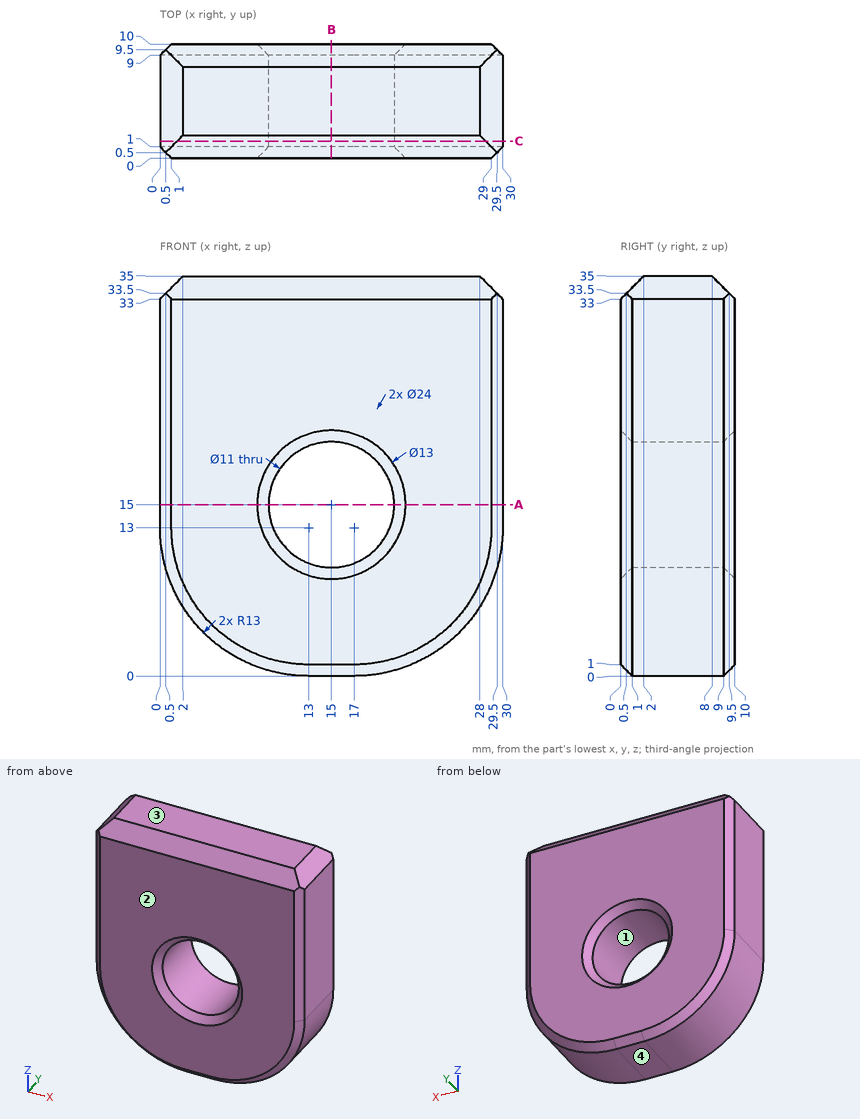
Job drawing, mm, ordinate dimensions from the low corner. One solid piece. Give positions to 0.01 mm unless a question says otherwise; leave off trailing zeros. Loops run counter-clockwise (first coordinate to the right, second up) from the corner with the lowest first, then second, coordinate; pieces in that order, holes last. Notation, with made-up numbers: (-19, 58.25) -> (3, 58.25) arc R25 cw to (3, 71.25) -> close; hole circle Ø3 at (85, 38). An arc over 180 degrees is marked (long way). Use a Markdown table: item, result. Add a question column.
(1) Wall check: line 1 along Z through (x, y) = (15, 3.75); line 2 along X through (y, z) = (4.5, 11.5); line 3 along X through (y, z) = (1.5, 17). Give the ranges that are in metal, low to high.
(2) Slice it at A-A on z = 15. List the corners of the cut face in (x, y).
(3) Mould opens along Z. For the marked faces 1, 2, 3 and 4 say: +Z half, -Z half, draft (parallel to the pull), parting line (faces both ways), or undercut.
(4) Slice it at B-B on x = 15. List the corners of the cut face in (y, z), and give its area (3 significant figures).
(5) Drop a flat-ended pin along its axis: pin 1 Ø1 at (y, z) = (3.5, 5.5) entering from +X. Give the stop position or say it passes through.
(6) Slice it at C-C on y = 1.5. List the corners of the cut face in (x, z).
Filled sheet:
| question | item | result |
|---|---|---|
| 1 | line 1 | 0 to 9.5, 20.5 to 35 |
| 1 | line 2 | 0.09 to 10.76, 19.24 to 29.91 |
| 1 | line 3 | 0 to 9.88, 20.12 to 30 |
| 2 | outline | (0, 1) -> (1, 0) -> (8.5, 0) -> (9.5, 1) -> (9.5, 9) -> (8.5, 10) -> (1, 10) -> (0, 9) -> close; (20.5, 1) -> (21.5, 0) -> (29, 0) -> (30, 1) -> (30, 9) -> (29, 10) -> (21.5, 10) -> (20.5, 9) -> close |
| 3 | face 1 | undercut |
| 3 | face 2 | draft |
| 3 | face 3 | +Z half |
| 3 | face 4 | -Z half |
| 4 | outline | (0, 1) -> (1, 0) -> (9, 0) -> (10, 1) -> (10, 8.5) -> (9, 9.5) -> (1, 9.5) -> (0, 8.5) -> close; (0, 21.5) -> (1, 20.5) -> (9, 20.5) -> (10, 21.5) -> (10, 33) -> (8, 35) -> (2, 35) -> (0, 33) -> close |
| 4 | area | 233 mm2 |
| 5 | pin 1 | x = 27.95 |
| 6 | outline | (0, 13) arc R13 ccw to (13, 0) -> (17, 0) arc R13 ccw to (30, 13) -> (30, 33) -> (28.5, 34.5) -> (1.5, 34.5) -> (0, 33) -> close; hole circle Ø11 at (15, 15) |
